Input: dimensioned drawing with shaded views. Units: mm. Origin: part minimum x, y, z. A direction names the side the tool comes from. Give positions to 0.01 mm unless a question says otherwise; leave off trailing zeros. Write each loop counter-clockwise with the first axis right and the second up, starting at its lowest first coordinate (ties: lowest second). Pieces come first, ordered by that corner, then holes. Notation, with made-up numbers: (-24.75, 47) -> (20.25, 47) arc R20 ccw to (20.25, 85) -> close; hole circle Ø6 at (56, 19). An arc over 180 degrees is marked (long way). Return JSON: item names as keys, results as strings. Group by question number.
Item 1: Section B-B, the plane y = 18.25. Return loops of the section in (x, z) (3 decimals).
Item 2: Pin query (flat end, axial travel): P1, Ø1, axis at x = 5, z = 1, coming from the +Y side. Return the tip coordinate at first contact, or that it passes through.
Item 3: Section A-A, the plane z = 2.6. Return loops of the section in (x, y) (3 decimals).
Item 4: Set-up query: the marked faces 1, 2 and 3. Return all of +Z, -Z, +X, -X, +Y, -Y with unobstructed straight access to the full face (end or side cutting, diameter ignored); none if empty.
Item 5: Section D-D, the plane y = 5. Return loops of the section in (x, z), then the cut area to 3 significant figures.
Item 6: Line query: line 1 (Y direction, x = 0.75, z = 1.85); line 2 (X direction, y = 18.75, z = 1.95); line 3 (X direction, y = 10.5, z = 4.8). Output: solid intervals per line, ascending. Write a range as [from, to].
Item 7: Section C-C, the plane x = 2. Return loops of the section in (y, z), then the cut area to 3 significant figures.
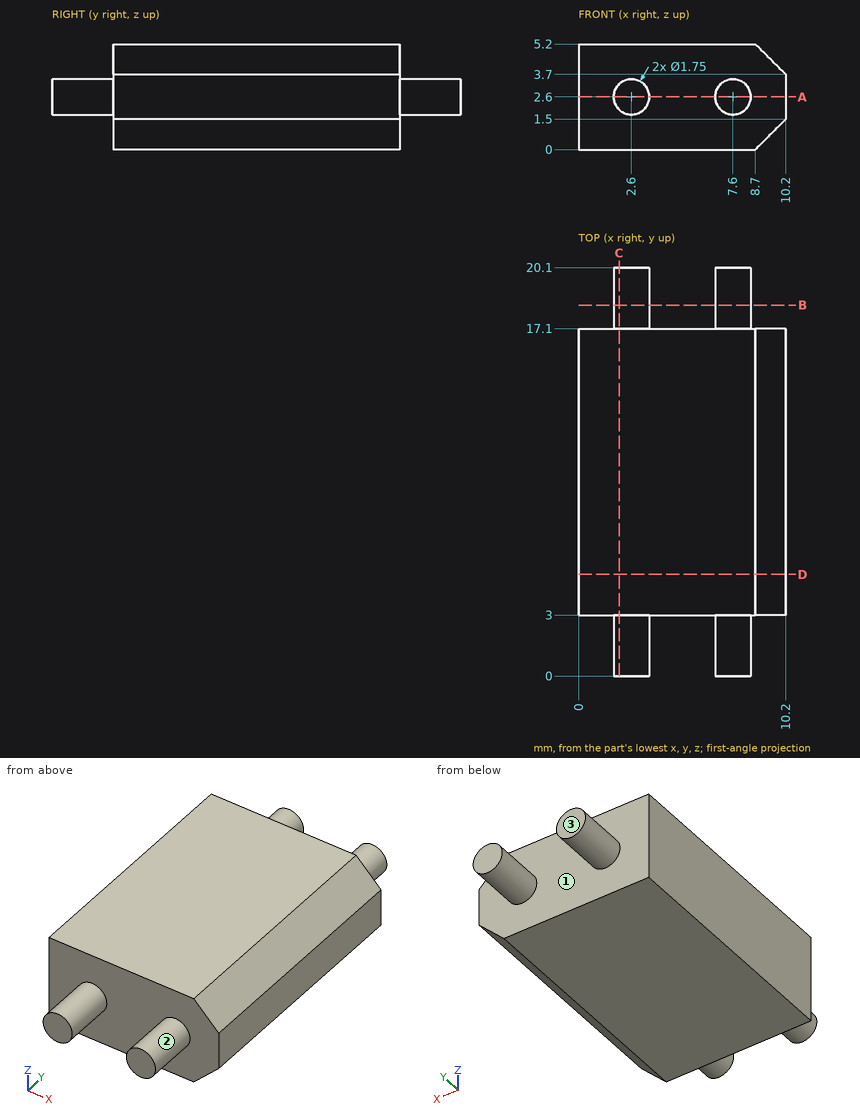
Answer below:
{
 "1": {"outline": "circle Ø1.75 at (2.6, 2.6); circle Ø1.75 at (7.6, 2.6)"},
 "2": {"P1": "stops at y = 17.1"},
 "3": {"outline": "(0, 3) -> (1.725, 3) -> (1.725, 0) -> (3.475, 0) -> (3.475, 3) -> (6.725, 3) -> (6.725, 0) -> (8.475, 0) -> (8.475, 3) -> (10.2, 3) -> (10.2, 17.1) -> (8.475, 17.1) -> (8.475, 20.1) -> (6.725, 20.1) -> (6.725, 17.1) -> (3.475, 17.1) -> (3.475, 20.1) -> (1.725, 20.1) -> (1.725, 17.1) -> (0, 17.1) -> close"},
 "4": {"face 1": "+Y", "face 2": "-Y", "face 3": "+Z, -Z, +X, -X, +Y"},
 "5": {"outline": "(0, 0) -> (8.7, 0) -> (10.2, 1.5) -> (10.2, 3.7) -> (8.7, 5.2) -> (0, 5.2) -> close", "area": "50.8 mm2"},
 "6": {"line 1": "y = [3, 17.1]", "line 2": "x = [2.01, 3.19], [7.01, 8.19]", "line 3": "x = [0, 9.1]"},
 "7": {"outline": "(0, 1.96) -> (3, 1.96) -> (3, 0) -> (17.1, 0) -> (17.1, 1.96) -> (20.1, 1.96) -> (20.1, 3.24) -> (17.1, 3.24) -> (17.1, 5.2) -> (3, 5.2) -> (3, 3.24) -> (0, 3.24) -> close", "area": "81.0 mm2"}
}
